Autodesk Fusion 360 part; units mm, degrees
sketch "Sketch1" plane through (0, 0, 0) normal (0, 0, 1) x (1, 0, 0) in component "link"
  line L0 (0, 0) -> (14, 0)
  line L1 (14, 0) -> (14, -14)
  line L2 (14, -14) -> (0, -14)
  line L3 (0, -14) -> (0, 0)
  circle A0 centre (7, -7) radius 5
  circle A1 centre (7, -7) radius 1.95
  dimension "d68" = 14
  dimension "d69" = 10
  dimension "d70" = 7
  dimension "d72" = 3.9
  dimension "d105" = 14
  dimension "d106" = 7
extrude "Extrude3" add sketch "Sketch1" along normal blind 6.5 contours L0 L1 L2 L3 | A0 | A1 in component "link"
extrude "Extrude4" cut sketch "Sketch1" along normal up to surface (6.5 mm away) contours A1 in component "link"
ref_plane "WorkPlane1" through (7, -7, 3.25) normal (1, 0, 0) x (0, 1, 0)
sketch "Sketch3" plane through (7, -7, 3.5) normal (1, 0, 0) x (0, 1, 0) in component "link"
  line L0 (0, 0) -> (14, 0) construction
  line L1 (14, 0) -> (14, 7) construction
  line L2 (14, 7) -> (0, 7)
  line L3 (0, 7) -> (0, 0) construction
  line L4 (5.5, 3.0262) -> (0, -0.9738)
  line L5 (0, -0.9738) -> (0, 3.0262)
  line L6 (0, 3.0262) -> (5.5, 3.0262)
  point P0 (7, 0)
  dimension "d109" = 5.5
  dimension "d110" = 4
revolve "Revolve1" cut sketch "Sketch3" angle 360 about axis through (7, -7, 10.5) along (0, 0, -1) in component "link"
fillet "Fillet2" radius 1 4 edges at (0, -14, 3.25) (0, 0, 3.25) (14, -14, 3.25) (14, 0, 3.25) in component "link"
component "link" placed x (1, 0, 0) y (0, 1, 0) z (0, 0, 1) at (0, 0, 0)
equation "ballJointHoleDim = 22.3 mm"
equation "tubeThickness = 2 mm"
equation "stockThickness = 9.6 mm"
equation "baseHeight = 5.5 mm"
equation "screwsCenterDistance = 32 mm"
equation "baseLength = 42 mm"
equation "ballJointBottomFromGround = 2 mm"
equation "screwHoleDiam = 3.5 mm"
equation "screwHeadHoleDiam = 6.3 mm"
equation "screwHeadHeight = 2 mm"
equation "ballJointHeight = 7 mm"
equation "linkStockHeight = 12.8 mm"
equation "linkWidth = 9.4 mm"
equation "linkHoleCenterDistance = 41 mm"
equation "linkBallJoinInsertDiam = 8.1 mm"
equation "linkBallInsertHeight = 6.8 mm"
equation "linkClearanceHeigt = 1 mm"
equation "toolDiameter = 2 mm"
Geometry check sheet. Reference: the model listing, model coordinates, mm. Coordinates: 2 decimals unless noted, no trailing zeros. Loops run counter-clockwise (first coordinate to the right, second up) from the corner with the lowest first, then second, coordinate; pieces in that order, holes last.
Item 1: Thickness scan on line 1 (X direction, y = -7, z = 3.15); line 2 (Y direction, x = 7, z = 1.65); line 3 (X direction, y = -10.5, z = 6). Record the ranges inside material, lowest first.
Item 2: Sectioned sample at B-B, the plane z = 3.75. Record the boundary of the cut face in (x, y), then the cut area to 3 significant figures.
Item 3: Release check for a two-part mould opening along X. For faces 1 (the face through (7, 0, 3)), 2 (the face through (5.052, -7.086, 1.945)), 3 (the face through (0.285, -13.699, 3.296)) record: released by +X, released by -X, zero draft, split by the parting line, or undercut.
Item 4: Sectioned sample at C-C, the plane z = 4.75. Record the boundary of the cut face in (x, y), then the cut area to 3 significant figures.
Item 5: Sectioned sample at A-A, the plane y = -7. Record the boundary of the cut face in (x, z).
Item 6: Go/stop test with a flat-tipped pin: pin 1 Ø6 at (x, y) = (7, -7) entering from +Z. Record where the tip stops, or that it passes through.
Check result:
1. line 1: x = 0 to 5.05, 8.95 to 14
1. line 2: y = -14 to -8.95, -5.05 to 0
1. line 3: x = 0 to 3.75, 10.25 to 14
2. outline: (0, -13) arc R1 ccw to (1, -14) - (13, -14) arc R1 ccw to (14, -13) - (14, -1) arc R1 ccw to (13, 0) - (1, 0) arc R1 ccw to (0, -1) - close; hole circle Ø3.9 at (7, -7)
2. area: 183 mm2
3. face 1: zero draft
3. face 2: undercut
3. face 3: released by -X
4. outline: (0, -13) arc R1 ccw to (1, -14) - (13, -14) arc R1 ccw to (14, -13) - (14, -1) arc R1 ccw to (13, 0) - (1, 0) arc R1 ccw to (0, -1) - close; hole circle Ø6.12 at (7, -7)
4. area: 166 mm2
5. outline: (0, 0) - (5.05, 0) - (5.05, 3.94) - (1.54, 6.5) - (0, 6.5) - close; (8.95, 0) - (14, 0) - (14, 6.5) - (12.46, 6.5) - (8.95, 3.94) - close
6. pin 1: stops at z = 4.71
